The model under review builds one solid part; all positions refer to its coordinate system, in mm. Round coordinates to 2 decimals unless told otherwise and drop trailing zeros. Write each loop counter-clockwise with the first axis right and the second up, starting at its lowest first coordinate (ties: lowest second). Pieces come first, ordered by that corner, then holes. Notation, with made-up numbers: M 24,-22.75 L 65,-22.75 A29 cw 65,0.25 Z; hole C 17.25,67 d9. An arc over 180 degrees is marked long. Write item = value, one per line. Start each with the question number.
Item 1: The part is to be moulded in two halves that separate along X. For faces 1 (the cylindrical face through (2.43, 11.85, 2.47)), 2 (the flat face through (77.4, 30, 2)), 3 (the flat face through (38, 0, 2)), say which applies: +X half, -X half, draft (parallel to the pull), parting line (faces both ways), or undercut.
Item 2: Take a section at A-A, the plane x = 73.4. Give the boundary of the cut face in (y, z).
Item 3: Take a section at B-B, the plane y = 21.5. Give the boundary of the cut face in (x, z), plus the area to 3 significant figures.
Item 4: Take a section at D-D, the plane z = 2.45. Give the boundary of the cut face in (x, y).
Item 5: To check wall thickness, follow line 1 along Y through (x, z) = (73.4, 3.75); line 2 along Y through (x, z) = (74, 2.6); line 3 along Y through (x, z) = (47.4, 2.75). State the ranges of each line that lie inside material, in increasing order.
Item 6: Take a section at C-C, the plane x = 47.4. Give the boundary of the cut face in (y, z), plus the area to 3 significant figures.
from build123d import *

# Parameters (mm, degrees)
SKETCH_1_W              = 77.4
SKETCH_1_H              = 60
EXTRUDE_1_DEPTH         = 5
SKETCH_2_R              = 17.5
CUT_EXTRUDE_1_DEPTH     = 99.059981644
HOLE_WIZARD_3_4_3_4_2_D = 3.4


with BuildPart() as part:
    # ｽｹｯﾁ1 → ﾎﾞｽ - 押し出し1 (new body)
    with BuildSketch(Plane.XY):
        with Locations((38.7, 30)):
            Rectangle(SKETCH_1_W, SKETCH_1_H)
    extrude(amount=EXTRUDE_1_DEPTH)

    # ｽｹｯﾁ2 → ｶｯﾄ - 押し出し1 (cut, through all)
    with BuildSketch(Plane.XY.offset(5)):
        with Locations((47.4, 30)):
            Circle(SKETCH_2_R)
    extrude(amount=-CUT_EXTRUDE_1_DEPTH, mode=Mode.SUBTRACT)

    # Ø3.4 (3.4) 直径の穴2 (through all)
    with Locations(Plane(origin=(73.4, 47.5, 5), x_dir=(1, 0, 0), z_dir=(0, 0, 1))):
        with Locations((0, 0), (0, -35), (-69.4, -35), (-69.4, 0)):
            Hole(HOLE_WIZARD_3_4_3_4_2_D / 2)


solid = part.part
Response values:
q1.face_1 = undercut
q1.face_2 = +X half
q1.face_3 = draft
q2.outline = M 0,0 L 10.8,0 L 10.8,5 L 0,5 Z; M 14.2,0 L 45.8,0 L 45.8,5 L 14.2,5 Z; M 49.2,0 L 60,0 L 60,5 L 49.2,5 Z
q3.outline = M 0,0 L 32.1,0 L 32.1,5 L 0,5 Z; M 62.7,0 L 77.4,0 L 77.4,5 L 62.7,5 Z
q3.area = 234 mm2
q4.outline = M 0,0 L 77.4,0 L 77.4,60 L 0,60 Z; hole C 4,12.5 d3.4; hole C 4,47.5 d3.4; hole C 47.4,30 d35; hole C 73.4,12.5 d3.4; hole C 73.4,47.5 d3.4
q5.line_1 = 0 to 10.8, 14.2 to 45.8, 49.2 to 60
q5.line_2 = 0 to 10.91, 14.09 to 45.91, 49.09 to 60
q5.line_3 = 0 to 12.5, 47.5 to 60
q6.outline = M 0,0 L 12.5,0 L 12.5,5 L 0,5 Z; M 47.5,0 L 60,0 L 60,5 L 47.5,5 Z
q6.area = 125 mm2
